The model under review builds one solid part; all positions refer to its coordinate system, in mm. A direction names the side the tool comes from. Give positions to 0.01 mm unless a question says otherwise; leave off trailing zeros. Loops run counter-clockwise (first coordinate to the right, second up) from the corner with the lowest first, then second, coordinate; pieces in that order, holes last. Notation, with made-up numbers: M -36,70 L -31,70 A8 ccw -31,81 Z; hole C -15,13.5 d10. An arc over 180 degrees is marked long. One line per item, written item: value. Start each with the question number.
Q1. To check wall thickness, follow line 1 along X through (y, z) = (8.5, -6.25); line 2 along Z through (x, y) = (4, 6.7); line 3 along Z through (x, y) = (4.5, 1.5). State the ranges of each line that lie inside material, in increasing order. Write a range as from..to.
Q2. We need section C-C on y = 0. Write out the cut boundary in (x, z).
Q3. We need section B-B on z = 0. Write out the cut boundary in (x, y).
Q4. Mouldability with a two-part tool opening along Y and no side actions: class faces 1 (the face through (4, -3, 0)), 2 (the face through (8, -9, -2)), 3 (the face through (-1.48, -10.74, -2.38)) as released by +Y, released by -Y, zero draft, split by the parting line, or undercut.
Q5. For faces 4 (the face through (0, 3.598, 0)), 5 (the face through (3.944, -8.786, 1.951)), 6 (the face through (5.386, 6.263, -0.575)), list the 3-axis set-ups (+Z, -Z, +X, -X, +Y, -Y) from which the entire face can be reached by the end or side of a thin tool; tool diameter is ignored.
Q6. For pin 1 (2.5 mm diameter, centred on x = 2, z = -0.5, fed in from -Y); pin 2 (0.7 mm diameter, centred on x = 1.5, y = 3.5, fed in from -Z); pin 3 (3.5 mm diameter, centred on x = 4, z = 0, fed in from +Y), all flat-tipped, find the tip position at first contact; note any pin that passes through.
Q7. We need section A-A on x = 7. Write out the cut boundary in (y, z).
Q8. We need section D-D on z = 9.5. Write out the cut boundary in (x, y), plus the area to 3 significant figures.
```python
from build123d import *

# Parameters (mm, degrees)
SKETCH1_R               = 9
BOSS_EXTRUDE1_DEPTH     = 8
SKETCH3_R               = 11
BOSS_EXTRUDE2_DEPTH     = 3
SKETCH4_R               = 11
BOSS_EXTRUDE3_DEPTH     = 3
CUT_EXTRUDE2_DEPTH      = 3
CUT_EXTRUDE2_DEPTH_BACK = 11
SKETCH6_R               = 1.5
CUT_EXTRUDE3_DEPTH      = 6


with BuildPart() as part:
    # Sketch1 → Boss-Extrude1 (new body)
    with BuildSketch(Plane(origin=(0, 0, 0), x_dir=(0, 0, -1), z_dir=(1, 0, 0))):
        Circle(SKETCH1_R)
    extrude(amount=BOSS_EXTRUDE1_DEPTH)

    # Sketch3 → Boss-Extrude2 (add)
    with BuildSketch(Plane(origin=(8, 0, 0), x_dir=(0, 0, -1), z_dir=(1, 0, 0))):
        Circle(SKETCH3_R)
    extrude(amount=BOSS_EXTRUDE2_DEPTH)

    # Sketch4 → Boss-Extrude3 (add)
    with BuildSketch(Plane.ZY):
        Circle(SKETCH4_R)
    extrude(amount=BOSS_EXTRUDE3_DEPTH)

    # Sketch2 → Cut-Extrude2 (cut, two sides)
    with BuildSketch(Plane(origin=(8, 0, 0), x_dir=(0, 0, -1), z_dir=(1, 0, 0))) as cut_extrude2_sk:
        with BuildLine():
            Line((-1.5, 3.598076211), (1.5, 3.598076211))
            Line((1.5, 3.598076211), (1.5, 2.711088342))
            ThreePointArc((1.5, 2.711088342), (1.525, 2.614263759), (1.59375, 2.541645321))
            ThreePointArc((1.59375, 2.541645321), (0, -3), (-1.59375, 2.541645321))
            ThreePointArc((-1.59375, 2.541645321), (-1.525, 2.614263759), (-1.5, 2.711088342))
            Line((-1.5, 2.711088342), (-1.5, 3.598076211))
        make_face()
    extrude(amount=CUT_EXTRUDE2_DEPTH, mode=Mode.SUBTRACT)
    extrude(cut_extrude2_sk.sketch, amount=-CUT_EXTRUDE2_DEPTH_BACK, mode=Mode.SUBTRACT)

    # Sketch6 → Cut-Extrude3 (cut)
    with BuildSketch(Plane.XZ.offset(-3.598076211)):
        with Locations((4, 0)):
            Circle(SKETCH6_R)
    extrude(amount=-CUT_EXTRUDE3_DEPTH, mode=Mode.SUBTRACT)


solid = part.part
```
Solved:
1. line 1: -3..0, 8..11
1. line 2: -6.01..-1.5, 1.5..6.01
1. line 3: -8.87..-2.6, 2.6..8.87
2. outline: M -3,-11 L 0,-11 L 0,-9 L 8,-9 L 8,-11 L 11,-11 L 11,-3 L -3,-3 Z; M -3,3 L 11,3 L 11,11 L 8,11 L 8,9 L 0,9 L 0,11 L -3,11 Z
3. outline: M -3,-11 L 0,-11 L 0,-9 L 8,-9 L 8,-11 L 11,-11 L 11,-3 L -3,-3 Z; M -3,3.6 L 2.5,3.6 L 2.5,9 L 0,9 L 0,11 L -3,11 Z; M 5.5,3.6 L 11,3.6 L 11,11 L 8,11 L 8,9 L 5.5,9 Z
4. face 1: undercut
4. face 2: zero draft
4. face 3: split by the parting line
5. face 4: +X, -X
5. face 5: none
5. face 6: +Y
6. pin 1: y = -9
6. pin 2: z = -8.43
6. pin 3: y = 9
7. outline: C 0,0 d18; hole M 2.54,-1.59 A0.2 cw 2.71,-1.5 L 3.6,-1.5 L 3.6,1.5 L 2.71,1.5 A0.2 cw 2.54,1.59 A3 ccw long Z
8. outline: M -3,-5.55 L 0,-5.55 L 0,5.55 L -3,5.55 Z; M 8,-5.55 L 11,-5.55 L 11,5.55 L 8,5.55 Z
8. area: 66.5 mm2
